```python
from build123d import *

# Parameters (mm, degrees)
SKETCH_1_R          = 2.25
EXTRUDE_1_DEPTH     = 0.3
SKETCH_2_R          = 1.5
EXTRUDE_3_DEPTH     = 24
SKETCH_6_R          = 1.75
EXTRUDE_4_DEPTH     = 0.1
DOME_1_FACE_RADIUS  = 1.75
DOME_1_HEIGHT       = 1
CUT_EXTRUDE_2_DEPTH = 2
CHAMFER_1_SIZE      = 0.2


with BuildPart() as part:
    # 草图1 → 凸台-拉伸1 (new body)
    with BuildSketch(Plane(origin=(0, 0, 0), x_dir=(0, 0, -1), z_dir=(1, 0, 0))):
        Circle(SKETCH_1_R)
    extrude(amount=EXTRUDE_1_DEPTH)

    # 草图2 → 凸台-拉伸3 (add)
    with BuildSketch(Plane.ZY):
        Circle(SKETCH_2_R)
    extrude(amount=EXTRUDE_3_DEPTH)

    # 草图6 → 凸台-拉伸4 (add)
    with BuildSketch(Plane(origin=(0.3, 0, 0), x_dir=(0, 0, -1), z_dir=(1, 0, 0))):
        Circle(SKETCH_6_R)
    extrude(amount=EXTRUDE_4_DEPTH)

    # 圆顶1: a dome of height H over a round flat face of radius A is a cap of a sphere of radius (A * A + H * H) / (2 * H)
    dome_1_r = (DOME_1_FACE_RADIUS * DOME_1_FACE_RADIUS + DOME_1_HEIGHT * DOME_1_HEIGHT) / (2 * DOME_1_HEIGHT)
    dome_1_base = Plane((0.4, 0, 0), z_dir=(1, 0, 0))
    with Locations(dome_1_base.offset(DOME_1_HEIGHT - dome_1_r)):
        dome_1_ball = Sphere(dome_1_r, mode=Mode.PRIVATE)
    add(split(dome_1_ball, bisect_by=dome_1_base, keep=Keep.TOP, mode=Mode.PRIVATE))

    # 草图5 → 切除-拉伸2 (cut)
    with BuildSketch(Plane(origin=(0, 0, 0), x_dir=(0, 0, -1), z_dir=(1, 0, 0))):
        Polygon((0.2, 0.2), (1.4, 0.2), (1.4, -0.2), (0.2, -0.2), (0.2, -1.4), (-0.2, -1.4), (-0.2, -0.2), (-1.4, -0.2), (-1.4, 0.2), (-0.2, 0.2), (-0.2, 1.4), (0.2, 1.4), align=None)
    extrude(amount=CUT_EXTRUDE_2_DEPTH, mode=Mode.SUBTRACT)

    # 倒角1
    chamfer_1_edges = [part.edges().sort_by_distance(p)[0] for p in [
        (-24, 0, -1.5),
    ]]
    chamfer(chamfer_1_edges, length=CHAMFER_1_SIZE)


solid = part.part
```
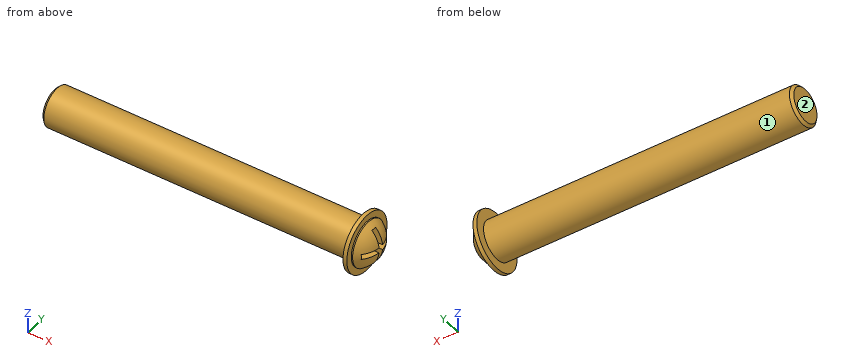
Source: CAD feature listing. Evaluate the final solid. Frame: model axes, mm. Face numbers are marked on the shaded views. A direction names the side the tool comes from. Give positions to 0.01 mm unless a question says otherwise; leave off trailing zeros. Order: outer loops, then holes, each group sorted by start corner. A loop starts at its lowest first (then second) coordinate and runs counter-clockwise, first axis right, second up.
(1) Section query A-A (x = -19.75). Return the cut outline in (y, z), plus the area to 3 significant figures.
(2) Access query for the marked faces 1 and 2. Directions: +Z, -Z, +X, -X, +Y, -Y. A direction counts if a zero-diameter tool reaches every point of the face in a straight line with its end or side. Return the directions, or none.
(3) Material intervals for line 1 along Z through (x, y) = (-6.5, -0.05); line 2 along Y through (x, z) = (-3, -0.55); line 3 along X through (y, z) = (0.4, -1.9), sorted ascending.
(4) Section query B-B (y = -2). Return the cut outline in (x, z).
(5) Contact query for flat-ended pins moving along their axis: P1, Ø0.6, axis at x = 1, z = 1, coming from the +Y side; P2, Ø1, axis at x = 1, y = -1, coming from the +Z side; P3, Ø2, axis at x = -17, y = 0.5, coming from the -Z side. Output: stop coordinate, or through.
Outcome:
1. outline: circle Ø3 at (0, 0)
1. area: 7.07 mm2
2. face 1: -X
2. face 2: +Z, -Z, -X, +Y, -Y
3. line 1: z = -1.5 to 1.5
3. line 2: y = -1.4 to 1.4
3. line 3: x = 0 to 0.3
4. outline: (0, -1.03) - (0.3, -1.03) - (0.3, 1.03) - (0, 1.03) - close
5. P1: stops at y = 1.23
5. P2: stops at z = 1.46
5. P3: stops at z = -1.5
